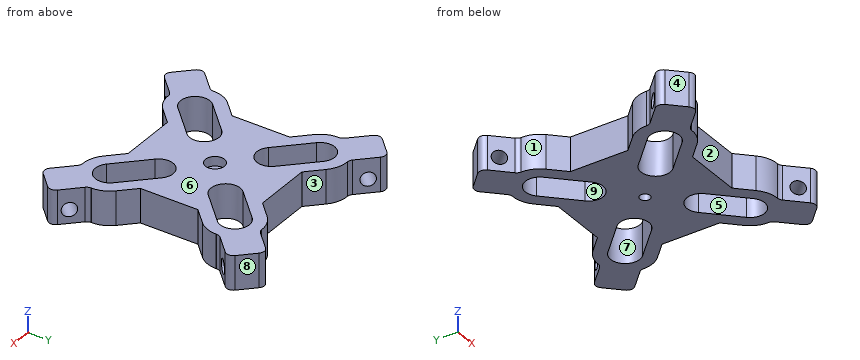
from build123d import *

# Parameters (mm, degrees)
SKETCH1_W                                      = 71.12
SKETCH1_H                                      = 71.12
EXTRUDE1_DEPTH                                 = 12.7
SKETCH3_R                                      = 2.921
CUT_EXTRUDE1_DEPTH                             = 13.7
MIRROR3_COPY_1_SKETCH_R                        = 2.921
MIRROR3_COPY_1_DEPTH                           = 13.7
MIRROR3_COPY_2_SKETCH_R                        = 2.921
MIRROR3_COPY_2_DEPTH                           = 13.7
SKETCH6_R                                      = 5.461
CUT_EXTRUDE3_DEPTH                             = 13.7
MIRROR6_COPY_1_SKETCH_R                        = 5.461
MIRROR6_COPY_1_DEPTH                           = 13.7
MIRROR6_COPY_2_SKETCH_R                        = 5.461
MIRROR6_COPY_2_DEPTH                           = 13.7
SKETCH7_W                                      = 71.12
SKETCH7_H                                      = 71.12
CUT_EXTRUDE5_DEPTH                             = 13.7
EXTRUDE2_DEPTH                                 = 12.7
CBORE_FOR_6_SOCKET_HEAD_CAP_SCREW1_D           = 3.7973
CBORE_FOR_6_SOCKET_HEAD_CAP_SCREW1_CBORE_D     = 7.14502
CBORE_FOR_6_SOCKET_HEAD_CAP_SCREW1_CBORE_DEPTH = 3.5052
MIRROR9_COPY_1_DEPTH                           = 12.7
FILLET3_R                                      = 2.54


with BuildPart() as part:
    # Sketch1 → Extrude1 (new body)
    with BuildSketch(Plane.XY):
        with Locations((-35.56, 35.56)):
            Rectangle(SKETCH1_W, SKETCH1_H)
    extrude(amount=EXTRUDE1_DEPTH)

    # Sketch3 → Cut-Extrude1 (cut, through all)
    with BuildSketch(Plane.XY.offset(12.7)):
        with Locations((-58.908665915, 58.908665915)):
            Circle(SKETCH3_R)
        with Locations((-48.132358569, 48.132358569)):
            Circle(SKETCH3_R)
        Polygon((-58.908665915, 58.908665915), (-56.843207007, 60.974124823), (-46.066899662, 50.197817477), (-50.197817477, 46.066899662), (-60.974124823, 56.843207007), align=None)
    cut_extrude1 = extrude(amount=-CUT_EXTRUDE1_DEPTH, mode=Mode.SUBTRACT)

    # Mirror1: Cut-Extrude1 across plane
    add(cut_extrude1.mirror(Plane.ZX.offset(35.56)), mode=Mode.SUBTRACT)

    # Mirror2: Cut-Extrude1 across plane
    add(cut_extrude1.mirror(Plane(origin=(-35.56, 0, 0), x_dir=(0, 0, 1), z_dir=(1, 0, 0))), mode=Mode.SUBTRACT)

    # Mirror3 copy 1 sketch → Mirror3 copy 1 (cut, through all)
    with BuildSketch(Plane(origin=(-71.12, 71.12, 12.7), x_dir=(-1, 0, 0), z_dir=(0, 0, 1))):
        with Locations((-58.908665915, 58.908665915)):
            Circle(MIRROR3_COPY_1_SKETCH_R)
        with Locations((-48.132358569, 48.132358569)):
            Circle(MIRROR3_COPY_1_SKETCH_R)
        Polygon((-58.908665915, 58.908665915), (-56.843207007, 60.974124823), (-46.066899662, 50.197817477), (-50.197817477, 46.066899662), (-60.974124823, 56.843207007), align=None)
    extrude(amount=-MIRROR3_COPY_1_DEPTH, mode=Mode.SUBTRACT)

    # Mirror3 copy 2 sketch → Mirror3 copy 2 (cut, through all)
    with BuildSketch(Plane(origin=(0, 71.12, 12.7), x_dir=(1, 0, 0), z_dir=(0, 0, 1))):
        with Locations((-58.908665915, -58.908665915)):
            Circle(MIRROR3_COPY_2_SKETCH_R)
        with Locations((-48.132358569, -48.132358569)):
            Circle(MIRROR3_COPY_2_SKETCH_R)
        Polygon((-58.908665915, -58.908665915), (-56.843207007, -60.974124823), (-46.066899662, -50.197817477), (-50.197817477, -46.066899662), (-60.974124823, -56.843207007), align=None)
    extrude(amount=-MIRROR3_COPY_2_DEPTH, mode=Mode.SUBTRACT)

    # Sketch6 → Cut-Extrude3 (cut, through all)
    with BuildSketch(Plane.XY.offset(12.7)):
        with Locations((-58.908665915, 58.908665915)):
            Circle(SKETCH6_R)
        with Locations((-48.132358569, 48.132358569)):
            Circle(SKETCH6_R)
        Polygon((-58.908665915, 58.908665915), (-55.047155783, 62.770176047), (-44.270848437, 51.993868702), (-48.132358569, 48.132358569), (-51.993868702, 44.270848437), (-62.770176047, 55.047155783), align=None)
    cut_extrude3 = extrude(amount=-CUT_EXTRUDE3_DEPTH, mode=Mode.SUBTRACT)

    # Mirror4: Cut-Extrude3 across plane
    add(cut_extrude3.mirror(Plane(origin=(-35.56, 0, 0), x_dir=(0, 0, 1), z_dir=(1, 0, 0))), mode=Mode.SUBTRACT)

    # Mirror5: Cut-Extrude3 across plane
    add(cut_extrude3.mirror(Plane.ZX.offset(35.56)), mode=Mode.SUBTRACT)

    # Mirror6 copy 1 sketch → Mirror6 copy 1 (cut, through all)
    with BuildSketch(Plane(origin=(-71.12, 71.12, 12.7), x_dir=(-1, 0, 0), z_dir=(0, 0, 1))):
        with Locations((-58.908665915, 58.908665915)):
            Circle(MIRROR6_COPY_1_SKETCH_R)
        with Locations((-48.132358569, 48.132358569)):
            Circle(MIRROR6_COPY_1_SKETCH_R)
        Polygon((-58.908665915, 58.908665915), (-55.047155783, 62.770176047), (-44.270848437, 51.993868702), (-48.132358569, 48.132358569), (-51.993868702, 44.270848437), (-62.770176047, 55.047155783), align=None)
    extrude(amount=-MIRROR6_COPY_1_DEPTH, mode=Mode.SUBTRACT)

    # Mirror6 copy 2 sketch → Mirror6 copy 2 (cut, through all)
    with BuildSketch(Plane(origin=(-71.12, 0, 12.7), x_dir=(-1, 0, 0), z_dir=(0, 0, 1))):
        with Locations((-58.908665915, -58.908665915)):
            Circle(MIRROR6_COPY_2_SKETCH_R)
        with Locations((-48.132358569, -48.132358569)):
            Circle(MIRROR6_COPY_2_SKETCH_R)
        Polygon((-58.908665915, -58.908665915), (-55.047155783, -62.770176047), (-44.270848437, -51.993868702), (-48.132358569, -48.132358569), (-51.993868702, -44.270848437), (-62.770176047, -55.047155783), align=None)
    extrude(amount=-MIRROR6_COPY_2_DEPTH, mode=Mode.SUBTRACT)

    # Sketch7 → Cut-Extrude5 (cut, through all)
    with BuildSketch(Plane.XY.offset(12.7)):
        with Locations((-35.56, 35.56)):
            Rectangle(SKETCH7_W, SKETCH7_H)
        with BuildLine():
            Line((-10.415282861, 24.783692655), (-5.027129188, 19.395538982))
            ThreePointArc((-5.027129188, 19.395538982), (-2.824718035, 16.099397758), (-2.051334085, 12.211334085))
            ThreePointArc((-2.051334085, 12.211334085), (-8.323270412, 2.824718035), (-19.395538982, 5.027129188))
            Line((-19.395538982, 5.027129188), (-24.783692655, 10.415282861))
            Line((-24.783692655, 10.415282861), (-46.336307345, 10.415282861))
            Line((-46.336307345, 10.415282861), (-51.724461018, 5.027129188))
            ThreePointArc((-51.724461018, 5.027129188), (-66.092870812, 5.027129188), (-66.092870812, 19.395538982))
            Line((-66.092870812, 19.395538982), (-60.704717139, 24.783692655))
            Line((-60.704717139, 24.783692655), (-60.704717139, 46.336307345))
            Line((-60.704717139, 46.336307345), (-66.092870812, 51.724461018))
            ThreePointArc((-66.092870812, 51.724461018), (-66.092870812, 66.092870812), (-51.724461018, 66.092870812))
            Line((-51.724461018, 66.092870812), (-46.336307345, 60.704717139))
            Line((-46.336307345, 60.704717139), (-24.783692655, 60.704717139))
            Line((-24.783692655, 60.704717139), (-19.395538982, 66.092870812))
            ThreePointArc((-19.395538982, 66.092870812), (-8.323270412, 68.295281965), (-2.051334085, 58.908665915))
            ThreePointArc((-2.051334085, 58.908665915), (-2.824718035, 55.020602242), (-5.027129188, 51.724461018))
            Line((-5.027129188, 51.724461018), (-10.415282861, 46.336307345))
            Line((-10.415282861, 46.336307345), (-10.415282861, 24.783692655))
        make_face(mode=Mode.SUBTRACT)
    extrude(amount=-CUT_EXTRUDE5_DEPTH, mode=Mode.SUBTRACT)

    # Sketch10 → Extrude2 (add)
    with BuildSketch(Plane.XY.offset(12.7)):
        Polygon((-68.786947648, 59.806691527), (-59.806691527, 68.786947648), (-68.786947648, 77.767203769), (-77.767203769, 68.786947648), align=None)
    extrude2 = extrude(amount=-EXTRUDE2_DEPTH)

    # CBORE for _6 Socket Head Cap Screw1 (through all)
    with Locations(Plane(origin=(-35.561282861, 35.558717139, 12.7), x_dir=(1, 0, 0), z_dir=(0, 0, 1))):
        with Locations((0, 0)):
            CounterBoreHole(CBORE_FOR_6_SOCKET_HEAD_CAP_SCREW1_D / 2, CBORE_FOR_6_SOCKET_HEAD_CAP_SCREW1_CBORE_D / 2, CBORE_FOR_6_SOCKET_HEAD_CAP_SCREW1_CBORE_DEPTH)

    # Sketch15 → 6 _0.204_ Diameter Hole1 (revolve, cut)
    with BuildSketch(Plane(origin=(-64.296819587, 73.277075708, 5.08), x_dir=(-0.707106781, 0.707106781, 0), z_dir=(0, 0, 1))):
        Polygon((0, 0), (0, 67.596709692), (2.5908, 66.04), (2.5908, 0), align=None)
    f_6_0_204_diameter_hole1 = revolve(axis=Axis((-59.806691527, 77.767203769, 5.08), (-0.707106781, -0.707106781, 0)), mode=Mode.SUBTRACT)

    # Mirror8: Extrude2, 6 _0.204_ Diameter Hole1 across plane
    add(extrude2.mirror(Plane.ZX.offset(35.56)))
    add(f_6_0_204_diameter_hole1.mirror(Plane.ZX.offset(35.56)), mode=Mode.SUBTRACT)

    # Mirror9: Extrude2, 6 _0.204_ Diameter Hole1 across plane
    add(extrude2.mirror(Plane(origin=(-35.56, 0, 0), x_dir=(0, 0, 1), z_dir=(1, 0, 0))))
    add(f_6_0_204_diameter_hole1.mirror(Plane(origin=(-35.56, 0, 0), x_dir=(0, 0, 1), z_dir=(1, 0, 0))), mode=Mode.SUBTRACT)

    # Mirror9 copy 1 sketch → Mirror9 copy 1 (add)
    with BuildSketch(Plane(origin=(-71.12, 71.12, 12.7), x_dir=(-1, 0, 0), z_dir=(0, 0, 1))):
        Polygon((-68.786947648, 59.806691527), (-59.806691527, 68.786947648), (-68.786947648, 77.767203769), (-77.767203769, 68.786947648), align=None)
    extrude(amount=-MIRROR9_COPY_1_DEPTH)

    # Mirror9 copy 2 sketch → Mirror9 copy 2 (revolve, cut)
    with BuildSketch(Plane(origin=(-6.823180413, -2.157075708, 5.08), x_dir=(0.707106781, -0.707106781, 0), z_dir=(0, 0, 1))):
        Polygon((0, 0), (0, 67.596709692), (2.5908, 66.04), (2.5908, 0), align=None)
    revolve(axis=Axis((-11.313308473, -6.647203769, 5.08), (0.707106781, 0.707106781, 0)), mode=Mode.SUBTRACT)

    # Fillet3
    fillet3_edges = [part.edges().sort_by_distance(p)[0] for p in [
        (-69.006962125, 60.026706004, 6.35),
        (-60.026706004, 69.006962125, 6.35),
        (-68.786947648, 77.767203769, 6.35),
        (-77.767203769, 68.786947648, 6.35),
        (-60.026706004, 2.113037875, 6.35),
        (-69.006962125, 11.093293996, 6.35),
        (-77.767203769, 2.333052352, 6.35),
        (-68.786947648, -6.647203769, 6.35),
        (-11.093293996, 69.006962125, 6.35),
        (-2.113037875, 60.026706004, 6.35),
        (6.647203769, 68.786947648, 6.35),
        (-2.333052352, 77.767203769, 6.35),
        (-2.113037875, 11.093293996, 6.35),
        (-11.093293996, 2.113037875, 6.35),
        (-2.333052352, -6.647203769, 6.35),
        (6.647203769, 2.333052352, 6.35),
    ]]
    fillet(fillet3_edges, radius=FILLET3_R)


solid = part.part
Could you check a few things on this model? Use its own coordinates, in mm. Face numbers are marked on the shaded views. A direction names the side the tool comes from. Coordinates: 2 decimals unless noted, no trailing zeros. Order: outer loops, then holes, each group sorted by start corner. A loop starts at its lowest first (then second) coordinate and runs counter-clockwise, first axis right, second up.
Q1. Thinking about a two-plate mould opening in Y: for the marked faces 6, 7, 8 and 9, which applies, released by +Y, released by -Y, zero draft, split by the parting line, or undercut?
Q2. Will these pins go through, and if not, where does the flat tip stop? pin 1 (4.5 mm diameter, centred on x = -35.56, y = 35.56, fed in from +Z); pin 2 (5 mm diameter, centred on x = -35, z = 8.5, fed in from -Y); pin 3 (5 mm diameter, centred on y = 31, z = 5.5, fed in from +X).
Q3. Please list where these lines run through material, in increasing order: L1, parallel to X at y = 9.5, z = 5.25; L2, parallel to Y at x = -25.5, z = 1.25; L3, parallel to Y at x = -52, z = 11.75.
Q4. Suppose I cut it at A-A on y = 49.5. Please give me the cut outline in (x, z).
Q5. Suppose I cut it at C-C on z = 6.25. Give the number of separate pieces and of enclosed holes in the cut face, and give its area (3 significant figures).
Q6. Which directions (+Z, -Z, +X, -X, +Y, -Y) give clear straight access to the entire face, cutting with the end or side of a thin tool? Please do the marked faces 1, 2, 3, 4 and 5.
Q7. Suppose I cut it at B-B on x = -17.5. Please give me the cut outline in (y, z), and give its area (3 significant figures).
Answer:
1. face 6: zero draft
1. face 7: undercut
1. face 8: released by +Y
1. face 9: undercut
2. pin 1: stops at z = 9.19
2. pin 2: stops at y = 10.42
2. pin 3: stops at x = -10.42
3. L1: x = -70.6 to -63.65, -53.9 to -47.25, -23.87 to -17.22, -7.47 to -0.52
3. L2: y = 10.42 to 17.78, 27.84 to 43.28, 53.34 to 60.7
3. L3: y = 4.76 to 11.4, 26.84 to 44.28, 59.72 to 66.36
4. outline: (-63.87, 0) - (-57.22, 0) - (-57.22, 12.7) - (-63.87, 12.7) - close; (-42.85, 0) - (-28.27, 0) - (-28.27, 12.7) - (-42.85, 12.7) - close; (-13.9, 0) - (-7.25, 0) - (-7.25, 12.7) - (-13.9, 12.7) - close
5. separate pieces: 5
5. enclosed holes: 5
5. area: 2,640 mm2
6. face 1: +Z, -Z, -X
6. face 2: +Z, -Z, -Y
6. face 3: +Z, -Z, +Y
6. face 4: +Z, -Z, -X, -Y
6. face 5: +Z, -Z
7. outline: (3.54, 0) - (9.78, 0) - (9.78, 12.7) - (3.54, 12.7) - close; (25.22, 0) - (45.9, 0) - (45.9, 12.7) - (25.22, 12.7) - close; (61.34, 0) - (67.58, 0) - (67.58, 12.7) - (61.34, 12.7) - close
7. area: 421 mm2
